Geometry check sheet. Reference: the model listing, model coordinates, mm. A direction names the side the tool comes from. Give positions to 0.01 mm unless a question says otherwise; leave off trailing zeros. Write each loop counter-clockwise with the first axis right and the second up, starting at its lowest first coordinate (ties: lowest second). Pieces come first, ordered by that corner, then holes. Notation, with made-up numbers: M 74.5,15 L 128.5,15 A12 cw 128.5,33 Z; hole C 2,63 d1. An arc over 180 degrees is marked long. Use one line per item in the form item = value. Start each with the question number.
Autodesk Inventor part; units mm, degrees
ref_plane "YZ Plane" through (0, 0, 0) normal (1, 0, 0) x (0, 1, 0)
ref_plane "XZ Plane" through (0, 0, 0) normal (0, 1, 0) x (-1, 0, 0)
ref_plane "XY Plane" through (0, 0, 0) normal (0, 0, 1) x (1, 0, 0)
sketch "Sketch1" plane through (0, 0, 0) normal (0, 1, 0) x (-1, 0, 0)
  line L0 (23.6, 14.625) -> (23.6, -14.625)
  line L1 (23.6, -14.625) -> (-10.25, -14.625)
  line L2 (-12.9, -14.125) -> (-12.9, -7.325)
  line L3 (-10.25, -6.825) -> (0, -6.825)
  line L4 (0, -6.825) -> (0, 6.825)
  line L5 (0, 6.825) -> (-10.25, 6.825)
  line L6 (-12.9, 7.325) -> (-12.9, 14.125)
  line L7 (-10.25, 14.625) -> (23.6, 14.625)
  line L8 (30.9, 0) -> (-20.2, 0)
  line L9 (-12.9, 14.125) -> (-10.25, 14.625)
  line L10 (-12.9, 7.325) -> (-10.25, 6.825)
  line L11 (-12.9, -7.325) -> (-10.25, -6.825)
  line L12 (-12.9, -14.125) -> (-10.25, -14.625)
  point P0 (-12.9, 6.825)
  point P1 (-12.9, 14.625)
  dimension "d0" = 29.25
  dimension "d1" = 23.6
  dimension "d2" = 7.8
  dimension "d3" = 12.9
  dimension "d14" = 6.825
  dimension "d15" = 13.65
  dimension "d16" = 6.8
  dimension "d17" = 6.8
  dimension "d18" = 2.65
  dimension "d19" = 2.65
  dimension "d20" = 2.65
  dimension "d21" = 2.65
  dimension "d22" = 0.5
  dimension "d23" = 0.5
extrude "Extrusion1" add sketch "Sketch1" along normal mid plane 0.8
sketch "Sketch2" plane through (0, 0, 0) normal (0, 1, 0) x (-1, 0, 0)
  line L0 (23.6, -14.625) -> (23.6, 14.625)
  line L1 (23.6, 14.625) -> (-10.25, 14.625)
  line L2 (0, 0) -> (0, -6.825)
  line L3 (0, 0) -> (0, 14.625)
  line L4 (0, -6.825) -> (0, -14.625)
  line L5 (-10.25, -14.625) -> (23.6, -14.625)
  point P0 (-12.9, 14.625)
extrude "Extrusion2" add sketch "Sketch2" along normal mid plane 9.15
sketch "Sketch3" plane through (0, -0.4, 14.625) normal (0, 0, 1) x (1, 0, 0)
  line L0 (-23.6, 4.975) -> (0, 4.975)
  line L1 (0, 0.8) -> (0, 4.975)
  line L2 (-5.2, 4.975) -> (0, 1.975)
  point P0 (0, 0.4)
  dimension "d10" = 5.2
  dimension "d11" = 3
extrude "Extrusion3" cut sketch "Sketch3" against normal blind 6
mirror "Mirror1" about plane through (0, 0, 0) normal (0, 0, 1) of "Extrusion3"
mirror "Mirror2" about plane through (0, 0, 0) normal (0, 1, 0) of "Extrusion3", "Mirror1"
equation "\"d14\" = 0.5 * d15"
properties part number "C0-1-01-circuitBreaker"
(1) Tool access check on faces 1 (the flat face through (7, 0.4, 11)), 2 (the flat face through (-1, 4, 8.625)), 3 (the flat face through (-1, -4, -8.625)). Record the directions out of +Z, -Z, +X, -X, +Y, -Y that give a thin tool (end or side, any length) a straight path to the whole face; none if there is none.
(2) Sectioned sample at C-C, the plane z = -9.5. Record the boundary of the cut face in (x, y) (3 decimals).
(3) Sectioned sample at A-A, the plane x = 7.5. Record the boundary of the cut face in (y, z) (3 decimals).
(4) Sectioned sample at D-D, the plane x = -2. Record the boundary of the cut face in (y, z) (3 decimals), plus the area to 3 significant figures.
(5) Depth check by flat-ended pin: pin 1 (0.9 mm diameter, centred on x = -1.5, y = 3, fed in from +Z) (3 decimals); pin 2 (3 mm diameter, centred on x = 9, y = 3, fed in from -Z); pin 3 (4 mm diameter, centred on x = 8.5, z = -10.5, fed in from +Y); pin 4 (4 mm diameter, centred on x = 5, z = 12.5, fed in from -Y). Enter the tip coordinate at first touch or a pass-through.
(6) Thickness scan on probe 1 along X at (y, z) = (-2.5, 5.25); probe 2 along Y at (x, z) = (3, -12.5); probe 3 along Z at (x, y) = (-1, -3.5) (3 decimals). Record the ranges inside material, lowest first. Write a range as [from, to].
(7) Sectioned sample at B-B, the plane y = 2.5. Record the boundary of the cut face in (x, z) (3 decimals), plus the area to 3 significant figures.
Numbers:
q1.face_1 = +Z, -Z, +X, +Y
q1.face_2 = +Z, +X, +Y
q1.face_3 = -Z, +X, -Y
q2.outline = M -23.6,-4.575 L -5.2,-4.575 L 0,-1.575 L 0,-0.4 L 12.9,-0.4 L 12.9,0.4 L 0,0.4 L 0,1.575 L -5.2,4.575 L -23.6,4.575 Z
q3.outline = M -0.4,-14.625 L 0.4,-14.625 L 0.4,-6.825 L -0.4,-6.825 Z; M -0.4,6.825 L 0.4,6.825 L 0.4,14.625 L -0.4,14.625 Z
q4.outline = M -4.575,-8.625 L -2.729,-8.625 L -2.729,-14.625 L 2.729,-14.625 L 2.729,-8.625 L 4.575,-8.625 L 4.575,8.625 L 2.729,8.625 L 2.729,14.625 L -2.729,14.625 L -2.729,8.625 L -4.575,8.625 Z
q4.area = 223 mm2
q5.pin_1 = 8.625
q5.pin_2 = through
q5.pin_3 = 0.4
q5.pin_4 = -0.4
q6.probe_1 = [-23.6, 0]
q6.probe_2 = [-0.4, 0.4]
q6.probe_3 = [-8.625, 8.625]
q7.outline = M -23.6,-14.625 L -1.603,-14.625 L -1.603,-8.625 L 0,-8.625 L 0,8.625 L -1.603,8.625 L -1.603,14.625 L -23.6,14.625 Z
q7.area = 671 mm2
